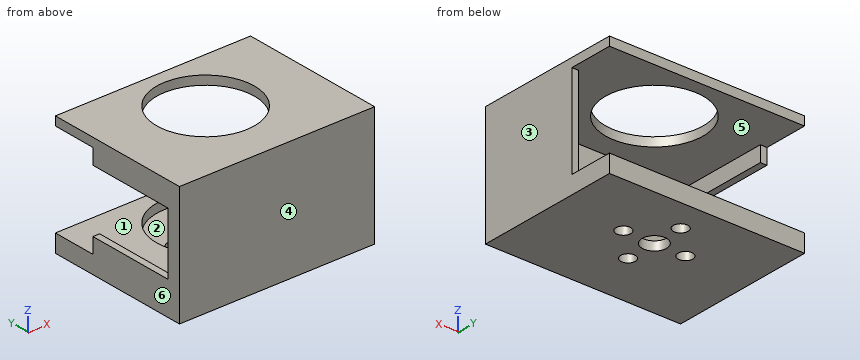
from build123d import *

# Parameters (mm, degrees)
SKETCH1_W               = 44
SKETCH1_H               = 27
BOSS_EXTRUDE1_DEPTH     = 23
CUT_EXTRUDE2_START      = 23
SKETCH2_W               = 41
SKETCH2_H               = 21
CUT_EXTRUDE2_DEPTH      = 20
CUT_EXTRUDE3_START      = -20.5
SKETCH3_W               = 14
SKETCH3_H               = 20
CUT_EXTRUDE3_DEPTH      = 20
BOSS_EXTRUDE2_START     = 23
SKETCH4_W               = 44
SKETCH4_H               = 4
SKETCH4_H_2             = 2
BOSS_EXTRUDE2_DEPTH     = 10
CUT_EXTRUDE4_DEPTH      = 42.895703837
CUT_EXTRUDE4_DEPTH_BACK = 2
CUT_EXTRUDE4_START      = -9.5
SKETCH5_R               = 11
CUT_EXTRUDE5_DEPTH      = 42.895703837
CUT_EXTRUDE5_DEPTH_BACK = 42.895703837
SKETCH6_R               = 1.65
SKETCH6_R_2             = 2.75


with BuildPart() as part:
    # Sketch1 → Boss-Extrude1 (new body)
    with BuildSketch(Plane(origin=(0, 0, 0), x_dir=(1, 0, 0), z_dir=(0, 1, 0))):
        Rectangle(SKETCH1_W, SKETCH1_H)
    extrude(amount=BOSS_EXTRUDE1_DEPTH)

    # Sketch2 → Cut-Extrude2 (cut)
    with BuildSketch(Plane(origin=(0, 0, 0), x_dir=(1, 0, 0), z_dir=(0, 1, 0)).offset(CUT_EXTRUDE2_START)):
        with Locations((0, -1)):
            Rectangle(SKETCH2_W, SKETCH2_H)
    extrude(amount=-CUT_EXTRUDE2_DEPTH, mode=Mode.SUBTRACT)

    # Sketch3 → Cut-Extrude3 (cut)
    with BuildSketch(Plane(origin=(0, 0, 0), x_dir=(0, 0, -1), z_dir=(1, 0, 0)).offset(CUT_EXTRUDE3_START)):
        with Locations((-1, 13)):
            Rectangle(SKETCH3_W, SKETCH3_H)
    extrude(amount=-CUT_EXTRUDE3_DEPTH, mode=Mode.SUBTRACT)

    # Sketch4 → Boss-Extrude2 (add)
    with BuildSketch(Plane(origin=(0, 0, 0), x_dir=(1, 0, 0), z_dir=(0, 1, 0)).offset(BOSS_EXTRUDE2_START)):
        with Locations((0, 11.5)):
            Rectangle(SKETCH4_W, SKETCH4_H)
        with Locations((0, -12.5)):
            Rectangle(SKETCH4_W, SKETCH4_H_2)
    extrude(amount=BOSS_EXTRUDE2_DEPTH)

    # Sketch5 → Cut-Extrude4 (cut, two sides: drawn at the far end of the back side and taken through both)
    with BuildSketch(Plane.XY.offset(CUT_EXTRUDE4_START - CUT_EXTRUDE4_DEPTH_BACK)):
        with Locations((0, 19)):
            Circle(SKETCH5_R)
    extrude(amount=CUT_EXTRUDE4_DEPTH + CUT_EXTRUDE4_DEPTH_BACK, mode=Mode.SUBTRACT)

    # Sketch6 → Cut-Extrude5 (cut, two sides: drawn at the far end of the back side and taken through both)
    with BuildSketch(Plane.XY.offset(-CUT_EXTRUDE5_DEPTH_BACK)):
        with Locations((-7, 19)):
            Circle(SKETCH6_R)
        with Locations((0, 19)):
            Circle(SKETCH6_R_2)
        with Locations((0, 26)):
            Circle(SKETCH6_R)
        with Locations((7, 19)):
            Circle(SKETCH6_R)
        with Locations((0, 12)):
            Circle(SKETCH6_R)
    extrude(amount=CUT_EXTRUDE5_DEPTH + CUT_EXTRUDE5_DEPTH_BACK, mode=Mode.SUBTRACT)


solid = part.part
Check sheet for the modelled part. Datum: model origin and axes. Units: mm. Face numbers are marked on the shaded views. A direction names the side the tool comes from. Coordinates: 2 decimals unless noted, no trailing zeros. Loops run counter-clockwise (first coordinate to the right, second up) from the corner with the lowest first, then second, coordinate; pieces in that order, holes last. Notation, with made-up numbers: (37, 33.5) -> (52, 33.5) arc R26 cw to (52, 57.5) -> close; hole circle Ø10 at (-30, 29). An arc over 180 degrees is marked (long way). Answer in a Markdown table with one row per item.
1. Release check for a two-part mould opening along X. For the marked faces 4, 5 and 6 record: released by +X, released by -X, zero draft, split by the parting line, or undercut.
Check values:
| item | result |
|---|---|
| face 4 | zero draft |
| face 5 | undercut |
| face 6 | released by -X |
2. Sectioned sample at C-C, the plane z = -7.5. Record the boundary of the cut face in (x, y), then the cut area to 3 significant figures.
Check values:
| item | result |
|---|---|
| outline | (-22, 0) -> (22, 0) -> (22, 23) -> (20.5, 23) -> (20.5, 3) -> (-20.5, 3) -> (-20.5, 23) -> (-22, 23) -> close |
| area | 192 mm2 |
3. Go/stop test with flat-tipped pins: pin 1 (4 mm diameter, centred on x = 0, y = 12, fed in from +Z); pin 2 (0.8 mm diameter, centred on x = -21.5, z = 10, fed in from +Y); pin 3 (5 mm diameter, centred on x = -15, z = 0, fed in from +Y); pin 4 (2.5 mm diameter, centred on x = 0, y = 26, fed in from -Z). Record where each tip stops, or that it passes through.
Check values:
| item | result |
|---|---|
| pin 1 | stops at z = -11.5 |
| pin 2 | stops at y = 23 |
| pin 3 | stops at y = 3 |
| pin 4 | passes through |
4. Material ranges on line 1 along X through (y, z) = (19, -12.95); line 2 along Y through (x, z) = (0, -12.95); line 3 along Z through (x, y) = (17, 7.5), recorded low to high. Write a range as [from, to].
Check values:
| item | result |
|---|---|
| line 1 | x = [-22, -8.65], [-5.35, -2.75], [2.75, 5.35], [8.65, 22] |
| line 2 | y = [0, 10.35], [13.65, 16.25], [21.75, 24.35], [27.65, 33] |
| line 3 | z = [-13.5, -9.5], [11.5, 13.5] |
5. Sectioned sample at A-A, the plane x = 0. Record the boundary of the cut face in (y, z).
Check values:
| item | result |
|---|---|
| outline | (0, -13.5) -> (10.35, -13.5) -> (10.35, -11.5) -> (8, -11.5) -> (8, -9.5) -> (3, -9.5) -> (3, 11.5) -> (8, 11.5) -> (8, 13.5) -> (0, 13.5) -> close; (13.65, -13.5) -> (16.25, -13.5) -> (16.25, -11.5) -> (13.65, -11.5) -> close; (21.75, -13.5) -> (24.35, -13.5) -> (24.35, -11.5) -> (21.75, -11.5) -> close; (27.65, -13.5) -> (33, -13.5) -> (33, -9.5) -> (30, -9.5) -> (30, -11.5) -> (27.65, -11.5) -> close; (30, 11.5) -> (33, 11.5) -> (33, 13.5) -> (30, 13.5) -> close |
6. Access from +Z, -Z, +X, -X, +Y, -Y to the whole of each face (thin tool, end or side, straight path). Record for the marked faces 1, 2 and 3.
Check values:
| item | result |
|---|---|
| face 1 | +Y |
| face 2 | +Z |
| face 3 | +Z, -Z, +X, +Y, -Y |
7. Sectioned sample at D-D, the plane y = 6. Record the boundary of the cut face in (x, z), then the cut area to 3 significant figures.
Check values:
| item | result |
|---|---|
| outline | (-22, -13.5) -> (22, -13.5) -> (22, 13.5) -> (-22, 13.5) -> (-22, 8) -> (-20.5, 8) -> (-20.5, 11.5) -> (20.5, 11.5) -> (20.5, -9.5) -> (-20.5, -9.5) -> (-20.5, -6) -> (-22, -6) -> close |
| area | 306 mm2 |
8. Sectioned sample at B-B, the plane y = 26. Record the boundary of the cut face in (x, z), then the cut area to 3 significant figures.
Check values:
| item | result |
|---|---|
| outline | (-22, -13.5) -> (-1.65, -13.5) -> (-1.65, -11.5) -> (-8.49, -11.5) -> (-8.49, -9.5) -> (-22, -9.5) -> close; (-22, 11.5) -> (-8.49, 11.5) -> (-8.49, 13.5) -> (-22, 13.5) -> close; (1.65, -13.5) -> (22, -13.5) -> (22, -9.5) -> (8.49, -9.5) -> (8.49, -11.5) -> (1.65, -11.5) -> close; (8.49, 11.5) -> (22, 11.5) -> (22, 13.5) -> (8.49, 13.5) -> close |
| area | 190 mm2 |
